Can you work these out from the model? Positions are in its coordinate system, mm. Give positions to 0.01 mm unless a question says otherwise; leave off trailing zeros. Write each loop counter-clockwise with the first axis right and the second up, starting at its lowest first coordinate (ties: lowest second). Pieces come first, ordered by that corner, then holes.
from build123d import *

# Parameters (mm, degrees)
SKETCH_1_W          = 150
SKETCH_1_H          = 145
SKETCH_1_R          = 1.6
SKETCH_1_W_2        = 2.916573318
SKETCH_1_H_2        = 67.038706503
EXTRUDE_1_DEPTH     = 4
SKETCH_2_R          = 2.1
SKETCH_2_R_2        = 1.6
CUT_EXTRUDE_1_DEPTH = 5
SKETCH_5_W          = 150
SKETCH_5_H          = 10
EXTRUDE_4_DEPTH     = 4
SKETCH_10_W         = 20
SKETCH_10_H         = 40
EXTRUDE_9_DEPTH     = 4
SKETCH_12_R         = 2.1
CUT_EXTRUDE_2_DEPTH = 5
SKETCH_15_W         = 50
SKETCH_15_H         = 20
SKETCH_15_R         = 1.6
EXTRUDE_11_DEPTH    = 4


with BuildPart() as part:
    # 草图1 → 凸台-拉伸1 (new body)
    with BuildSketch(Plane(origin=(0, 0, 0), x_dir=(1, 0, 0), z_dir=(0, 1, 0))):
        with Locations((0, -2.5)):
            Rectangle(SKETCH_1_W, SKETCH_1_H)
        with Locations((-20, 50)):
            Circle(SKETCH_1_R, mode=Mode.SUBTRACT)
        with Locations((20, 50)):
            Circle(SKETCH_1_R, mode=Mode.SUBTRACT)
        with Locations((-20, 35)):
            Circle(SKETCH_1_R, mode=Mode.SUBTRACT)
        with Locations((20, 35)):
            Circle(SKETCH_1_R, mode=Mode.SUBTRACT)
        with Locations((-46, 0)):
            Circle(SKETCH_1_R, mode=Mode.SUBTRACT)
        with Locations((24, 0)):
            Circle(SKETCH_1_R, mode=Mode.SUBTRACT)
        with Locations((24, 64.8)):
            Circle(SKETCH_1_R, mode=Mode.SUBTRACT)
        with Locations((40, -5)):
            Circle(SKETCH_1_R, mode=Mode.SUBTRACT)
        with Locations((40, -65)):
            Circle(SKETCH_1_R, mode=Mode.SUBTRACT)
        with Locations((56.637514727, -9.301063596)):
            Rectangle(SKETCH_1_W_2, SKETCH_1_H_2, mode=Mode.SUBTRACT)
    extrude(amount=EXTRUDE_1_DEPTH)

    # 草图2 → 切除-拉伸1 (cut, through all)
    with BuildSketch(Plane(origin=(0, 4, 0), x_dir=(1, 0, 0), z_dir=(0, 1, 0))):
        with Locations((0, -67)):
            Circle(SKETCH_2_R)
        with Locations((-66.052318668, 65)):
            Circle(SKETCH_2_R_2)
        with Locations((-66.052318668, 35)):
            Circle(SKETCH_2_R_2)
        with Locations((-42.052318668, 65)):
            Circle(SKETCH_2_R_2)
        with Locations((-42.052318668, 35)):
            Circle(SKETCH_2_R_2)
        with Locations((42.052318668, 35)):
            Circle(SKETCH_2_R_2)
        with Locations((66.052318668, 35)):
            Circle(SKETCH_2_R_2)
        with Locations((66.052318668, 65)):
            Circle(SKETCH_2_R_2)
        with Locations((42.052318668, 65)):
            Circle(SKETCH_2_R_2)
    extrude(amount=-CUT_EXTRUDE_1_DEPTH, mode=Mode.SUBTRACT)

    # 草图5 → 凸台-拉伸4 (add)
    with BuildSketch(Plane(origin=(0, 4, 0), x_dir=(1, 0, 0), z_dir=(0, 1, 0))):
        with Locations((0, -80)):
            Rectangle(SKETCH_5_W, SKETCH_5_H)
    extrude(amount=-EXTRUDE_4_DEPTH)

    # 草图10 → 凸台-拉伸9 (add)
    with BuildSketch(Plane.XZ):
        with Locations((-65, 105)):
            Rectangle(SKETCH_10_W, SKETCH_10_H)
        with Locations((65, 105)):
            Rectangle(SKETCH_10_W, SKETCH_10_H)
    extrude(amount=-EXTRUDE_9_DEPTH)

    # 草图12 → 切除-拉伸2 (cut, through all)
    with BuildSketch(Plane(origin=(0, 4, 0), x_dir=(1, 0, 0), z_dir=(0, 1, 0))):
        with Locations((-65, -113)):
            Circle(SKETCH_12_R)
        with Locations((65, -113)):
            Circle(SKETCH_12_R)
    extrude(amount=-CUT_EXTRUDE_2_DEPTH, mode=Mode.SUBTRACT)

    # 草图15 → 凸台-拉伸11 (add)
    with BuildSketch(Plane(origin=(0, 4, 0), x_dir=(1, 0, 0), z_dir=(0, 1, 0))):
        with Locations((100, -115)):
            Rectangle(SKETCH_15_W, SKETCH_15_H)
        with Locations((117, -115)):
            Circle(SKETCH_15_R, mode=Mode.SUBTRACT)
        with Locations((-100, -115)):
            Rectangle(SKETCH_15_W, SKETCH_15_H)
        with Locations((-117, -115)):
            Circle(SKETCH_15_R, mode=Mode.SUBTRACT)
    extrude(amount=-EXTRUDE_11_DEPTH)


solid = part.part
(1) Imagine slicing it at A-A, the plane z = 89.5. Write out the boundary of the cut face in (x, y).
Returned:
outline: (-75, 0) - (-55, 0) - (-55, 4) - (-75, 4) - close; (55, 0) - (75, 0) - (75, 4) - (55, 4) - close
(2) If I drill on L1, parallel to Z at x = 20, y = 1.75; L2, parallel to Z at x = 40, y = 3.1; L3, parallel to X at y = 1.6, z = -64.8, over which ranges is the centre line in solid material (lowest first)?
Returned:
L1: z = -70 to -51.6, -48.4 to -36.6, -33.4 to 85
L2: z = -70 to 3.4, 6.6 to 63.4, 66.6 to 85
L3: x = -75 to -67.64, -64.46 to -43.64, -40.46 to 22.4, 25.6 to 40.46, 43.64 to 64.46, 67.64 to 75
(3) Will these pins go through, and if not, where does the flat tip stop? P1, Ø3, axis at x = 66.05, z = -35, coming from the +Y side; P2, Ø1.2, axis at y = 2.5, z = -6, coming from the +X side; P3, Ø1, axis at x = -36, y = 3, coming from the +Z side; P4, Ø2, axis at y = 2.5, z = -17.5, coming from the -X side.
Returned:
P1: passes through
P2: stops at x = 75
P3: stops at z = 85
P4: stops at x = -75
(4) Imagine slicing it at C-C, the plane x = -80. Write out the boundary of the cut face in (y, z), plus the area to 3 significant figures.
Returned:
outline: (0, 105) - (4, 105) - (4, 125) - (0, 125) - close
area: 80.0 mm2
(5) Imagine slicing it at D-D, the plane y = 2.35. Give the number of separate pieces and of enclosed holes in the cut face, plus the area to 3 significant figures.
Returned:
separate pieces: 1
enclosed holes: 23
area: 26,500 mm2
(6) Imagine slicing it at B-B, the plane z = 26.5. Write out the boundary of the cut face in (x, y), plus the area to 3 significant figures.
Returned:
outline: (-75, 0) - (55.18, 0) - (55.18, 4) - (-75, 4) - close; (58.1, 0) - (75, 0) - (75, 4) - (58.1, 4) - close
area: 588 mm2
